The listing builds one solid part. Answer for the finished solid, in the listing's coordinates (mm). Face numbers are marked on the shaded views. Give positions to 0.01 mm unless a question says otherwise; leave off trailing zeros. Order: outer loops, then holes, each group sorted by start corner. A loop starts at its lowest first (then second) coordinate and runs counter-clockwise, first axis right, second up. Notation, with made-up numbers: (-6.75, -34) - (38.25, -34) arc R24 cw to (38.25, 2) - close; hole circle Ø11 at (11.5, 0.25). An arc over 180 degrees is marked (long way). Answer as a JSON object with one key per item and string values. Group by question number.
Q1. The mould has two halves that part along X. Classify the marked faces 1, 2 and 3: released by +X, released by -X, zero draft, split by the parting line, or undercut.
Q2. Given pin 1 (3 mm diameter, centred on x = 65.5, y = -43, fed in from +Z), flat-ended and moving along its own axis, determine where the tip first touches the part or whether it passes through.
Q3. Consider line 1 (Y direction, x = 75, z = 3); line 2 (X direction, y = -44.5, z = 6.75); line 3 (Z direction, x = 68.5, y = -41.25). Determine where each line is inside the solid, lowest interval first.
Q4. A cutting plane is placed at B-B, the plane z = 11. Give the vertices of the cut face in (x, y), and give its area (3 significant figures).
from build123d import *

# Parameters (mm, degrees)
F0_W     = 160
F0_H     = 25
F1_DEPTH = 15
F2_T     = -1
F3_R     = 0.5
F4_R     = 0.5
F5_R     = 0.49999


# Not quite as in the source:
# - a fillet or chamfer is up to 0.001 mm smaller than in the source, because OpenCascade refuses the exact size


with BuildPart() as f1:
    # F0 (on Top) → F1 (new body)
    with BuildSketch(Plane.XY):
        with Locations((30.8671402, -38.0363363773)):
            Rectangle(F0_W, F0_H)
    extrude(amount=F1_DEPTH)

    # F2
    f2_openings = [f1.faces().sort_by_distance(p)[0] for p in [
        (30.86714, -38.036336, 15),
    ]]
    offset(amount=F2_T, openings=f2_openings)

    # F3
    f3_edges = [f1.edges().sort_by_distance(p)[0] for p in [
        (30.86714, -25.536336, 0),
        (110.86714, -38.036336, 0),
        (-49.13286, -38.036336, 0),
        (30.86714, -50.536336, 0),
        (110.86714, -25.536336, 7.5),
        (-49.13286, -25.536336, 7.5),
        (-49.13286, -50.536336, 7.5),
        (110.86714, -50.536336, 7.5),
    ]]
    fillet(f3_edges, radius=F3_R)

    # F4
    f4_edges = [f1.edges().sort_by_distance(p)[0] for p in [
        (-48.13286, -38.036336, 1),
        (30.86714, -26.536336, 1),
        (30.86714, -49.536336, 1),
        (109.86714, -38.036336, 1),
        (-48.13286, -26.536336, 8),
        (-48.13286, -49.536336, 8),
        (109.86714, -26.536336, 8),
        (109.86714, -49.536336, 8),
    ]]
    fillet(f4_edges, radius=F4_R)

    # F5 (radius 0.5 in the source; OpenCascade refuses exactly that, so slightly less here)
    f5_edges = [f1.edges().sort_by_distance(p)[0] for p in [
        (30.86714, -25.536336, 15),
        (30.86714, -26.536336, 15),
        (30.86714, -49.536336, 15),
        (30.86714, -50.536336, 15),
        (109.86714, -38.036336, 15),
        (110.86714, -38.036336, 15),
        (-49.13286, -38.036336, 15),
        (-48.13286, -38.036336, 15),
        (-47.986413, -49.38989, 15),
        (-47.986413, -26.682783, 15),
        (-48.986413, -25.682783, 15),
        (-48.986413, -50.38989, 15),
        (109.720694, -26.682783, 15),
        (110.720694, -25.682783, 15),
        (109.720694, -49.38989, 15),
        (110.720694, -50.38989, 15),
    ]]
    fillet(f5_edges, radius=F5_R)


solid = f1.part
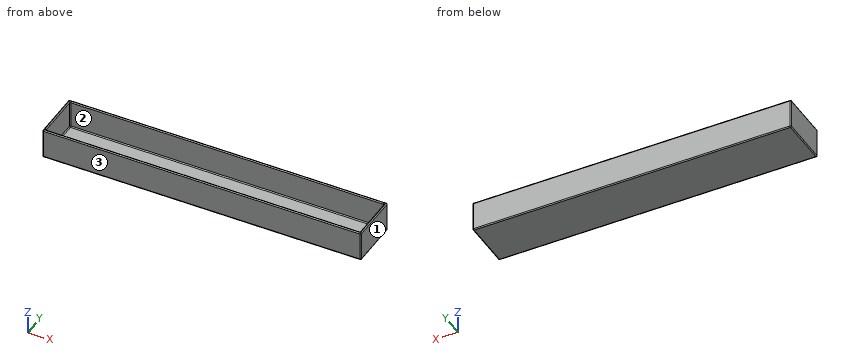
Reply:
{
 "1": {"face 1": "released by +X", "face 2": "undercut", "face 3": "zero draft"},
 "2": {"pin 1": "stops at z = 1"},
 "3": {"line 1": "y = -50.54 to -49.54, -26.54 to -25.54", "line 2": "x = -49.13 to -48.13, 109.87 to 110.87", "line 3": "z = 0 to 1"},
 "4": {"outline": "(-49.13, -50.04) arc R0.5 ccw to (-48.63, -50.54) - (110.37, -50.54) arc R0.5 ccw to (110.87, -50.04) - (110.87, -26.04) arc R0.5 ccw to (110.37, -25.54) - (-48.63, -25.54) arc R0.5 ccw to (-49.13, -26.04) - close; hole (-48.13, -49.04) arc R0.5 ccw to (-47.63, -49.54) - (109.37, -49.54) arc R0.5 ccw to (109.87, -49.04) - (109.87, -27.04) arc R0.5 ccw to (109.37, -26.54) - (-47.63, -26.54) arc R0.5 ccw to (-48.13, -27.04) - close", "area": "366 mm^2"}
}
